from build123d import *

# Parameters (mm, degrees)
SZKIC2_R                    = 20
SZKIC2_R_2                  = 15
SZKIC2_R_3                  = 11
SZKIC2_R_4                  = 6
DODANIE_WYCI_GNI_CIE2_DEPTH = 20


with BuildPart() as part:
    # Szkic2 → Dodanie-wyciągnięcie2 (new body)
    with BuildSketch(Plane.XY):
        with BuildLine():
            ThreePointArc((18.800305478, -6.822647135), (11.479265162, -16.377621053), (0, -20))
            Line((0, -20), (29.733250719, -20))
            Line((29.733250719, -20), (113.904224342, -9.156501468))
            ThreePointArc((113.904224342, -9.156501468), (109.006471259, -0.377260954), (113.290863107, 8.71707991))
            Line((113.290863107, 8.71707991), (27.069867273, 20))
            Line((27.069867273, 20), (0, 20))
            ThreePointArc((0, 20), (11.479265162, 16.377621053), (18.800305478, 6.822647135))
            Line((18.800305478, 6.822647135), (20.410663052, 9.615363763))
            Line((20.410663052, 9.615363763), (83.386650307, 3.862118667))
            ThreePointArc((83.386650307, 3.862118667), (88.740074522, -0.948230099), (82.9809258, -5.26457254))
            Line((82.9809258, -5.26457254), (20.107259976, -10.897738547))
            Line((20.107259976, -10.897738547), (18.800305478, -6.822647135))
        make_face()
        Circle(SZKIC2_R)
        Circle(SZKIC2_R_2, mode=Mode.SUBTRACT)
        with Locations((120, 0)):
            Circle(SZKIC2_R_3)
        with Locations((120, 0)):
            Circle(SZKIC2_R_4, mode=Mode.SUBTRACT)
    extrude(amount=DODANIE_WYCI_GNI_CIE2_DEPTH)


solid = part.part
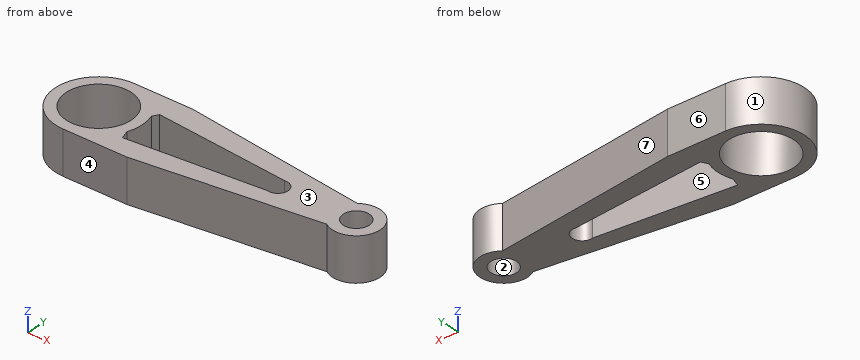
Work out the finished part from the listing and answer in its coordinate system (mm). Face numbers are marked on the shaded views. A direction names the side the tool comes from. Round coordinates to 2 decimals unless told otherwise and drop trailing zeros. Write each loop counter-clockwise with the first axis right and the second up, starting at its lowest first coordinate (ties: lowest second). Pieces come first, ordered by that corner, then holes. Notation, with made-up numbers: M 26.25,-16 L 32.25,-16 A18 ccw 32.25,17 Z; hole C -22.75,22 d3. An arc over 180 degrees is marked long. Use a Markdown table: item, result.
1) The part is cut by section D-D on x = 25.5. Give the vertices of the cut face in (y, z).
Taken from the geometry:
| item | result |
|---|---|
| outline | M -20,0 L -10.41,0 L -10.41,20 L -20,20 Z; M 9.15,0 L 20,0 L 20,20 L 9.15,20 Z |
2) The part is cut by section C-C on y = 1.5. Give the vertices of the cut face in (x, z).
Taken from the geometry:
| item | result |
|---|---|
| outline | M -19.94,0 L -14.92,0 L -14.92,20 L -19.94,20 Z; M 14.92,0 L 19.94,0 L 19.94,20 L 14.92,20 Z; M 88.17,0 L 114.19,0 L 114.19,20 L 88.17,20 Z; M 125.81,0 L 130.9,0 L 130.9,20 L 125.81,20 Z |
3) Which of the six approach directions +Z, -Z, +X, -X, +Y, -Y give full straight-line access (tool end or side, diameter ignored) to the marked faces 5, 6 and 7?
Taken from the geometry:
| item | result |
|---|---|
| face 5 | +Z, -Z |
| face 6 | +Z, -Z, +X, -X, +Y |
| face 7 | +Z, -Z, +Y |
4) Flat-ended cylindrical pins translate along their axes: pin 1 (2 mm diameter, centred on y = -7.5, z = 17, fed in from -X); pin 2 (10 mm diameter, centred on y = 12, z = 9.5, fed in from +X); pin 3 (4 mm diameter, centred on x = 40, z = 4, fed in from +Y). Find the tip coordinate at first contact, or state that the pin passes through.
Taken from the geometry:
| item | result |
|---|---|
| pin 1 | stops at x = -18.91 |
| pin 2 | stops at x = 128.49 |
| pin 3 | stops at y = 18.57 |
5) Determine the mould class of the marked faces 1, 2, 3 and 4 for opening direction Y: pulls with the +Y half, pulls with the -Y half, needs draft (parallel to the pull), parting line crosses it, or undercut.
Taken from the geometry:
| item | result |
|---|---|
| face 1 | parting line crosses it |
| face 2 | undercut |
| face 3 | needs draft |
| face 4 | pulls with the -Y half |
6) The part is cut by section A-A on x = 120. Give the vertices of the cut face in (y, z), plus the area to 3 significant figures.
Taken from the geometry:
| item | result |
|---|---|
| outline | M -11,0 L -6,0 L -6,20 L -11,20 Z; M 6,0 L 11,0 L 11,20 L 6,20 Z |
| area | 200 mm2 |
7) The part is cut by section B-B on z = 2. Give the vertices of the cut face in (x, y), plus the area to 3 significant figures.
Taken from the geometry:
| item | result |
|---|---|
| outline | M 0,-20 L 29.73,-20 L 113.9,-9.16 A11 ccw long 113.29,8.72 L 27.07,20 L 0,20 A20 ccw Z; hole C 0,0 d30; hole M 18.8,-6.82 L 20.11,-10.9 L 82.98,-5.26 A4.66 ccw long 83.39,3.86 L 20.41,9.62 L 18.8,6.82 A20 cw Z; hole C 120,0 d12 |
| area | 2,740 mm2 |
8) Consider line 1 (Y direction, x = 0, z = 1.75); line 2 (Y direction, x = 120, z = 4.5); line 3 (X direction, y = -2, z = 15.5). Determine where each line is inside the solid, lowest interval first. Write a range as [from, to].
Taken from the geometry:
| item | result |
|---|---|
| line 1 | y = [-20, -15], [15, 20] |
| line 2 | y = [-11, -6], [6, 11] |
| line 3 | x = [-19.9, -14.87], [14.87, 19.9], [88.57, 114.34], [125.66, 130.82] |
